Design review of the part shown in the three views and the two pictorial views. Dimensions are in mm from the part's minimum x, y and z. A direction names the side the tool comes from. Round coordinates to 2 decimals unless told otherwise and drop trailing zeros.
1) Tool access review of the marked faces 1, 2, 3 and 4: name each direction out of +Z, -Z, +X, -X, +Y, -Y from which nothing blocks a thin tool from reaching the whole face with its end or side.
2) Wall thickness on L1, parallel to Y at x = 0.9, z = 2.35; L2, parallel to X at y = 5.75, z = 1.7: over which ranges is each line inside the solid? List them lowest first.
3) Mouldability with a two-part tool opening along Y and no side actions: class the marked faces 5, 6 and 7 as pulls with the +Y half, pulls with the -Y half, needs draft (parallel to the pull), parting line crosses it, or undercut.
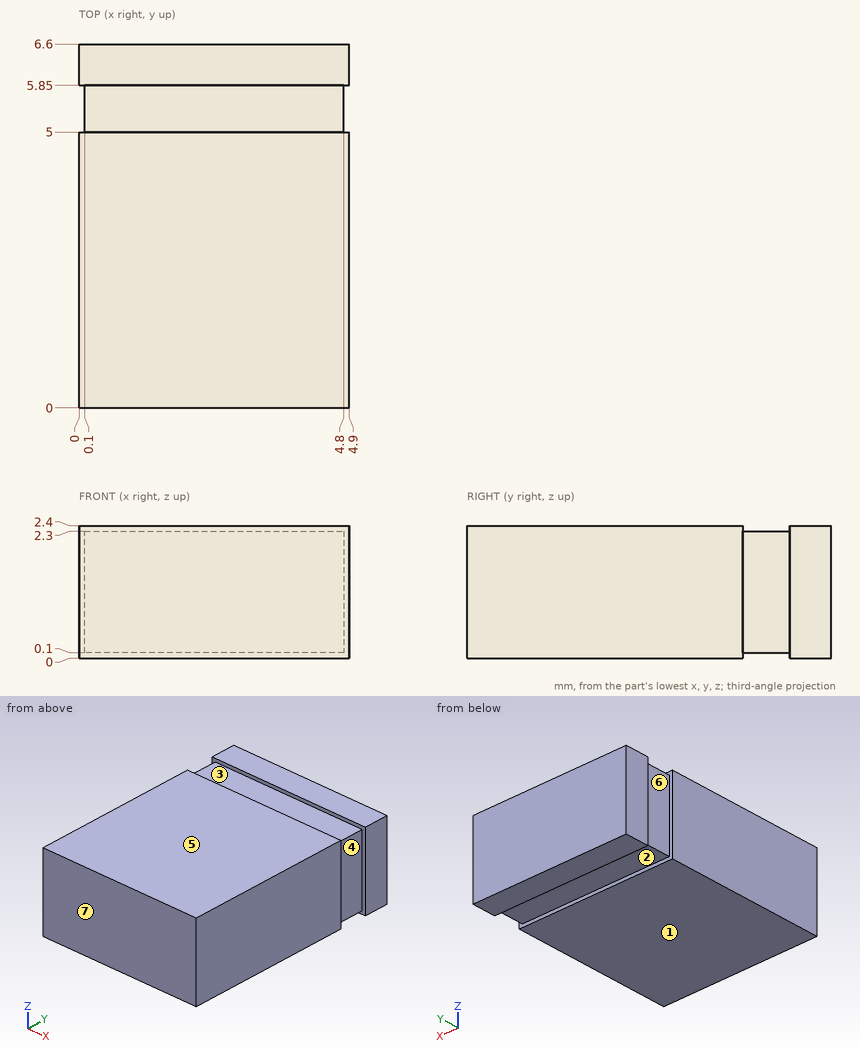
Response:
1. face 1: -Z, +X, -X, +Y, -Y
1. face 2: -Z, +X, -X
1. face 3: +Z, +X, -X
1. face 4: +Z, -Z, +X
2. L1: y = 0 to 5, 5.85 to 6.6
2. L2: x = 0.1 to 4.8
3. face 5: needs draft
3. face 6: undercut
3. face 7: pulls with the -Y half
